```python
from build123d import *

# Parameters (mm, degrees)
SKETCH1_R           = 5
BOSS_EXTRUDE1_DEPTH = 32
SKETCH1_4_R         = 7.5
SKETCH1_4_R_2       = 5
BOSS_EXTRUDE2_DEPTH = 5
BOSS_EXTRUDE3_START = 27
SKETCH1_5_R         = 7.5
SKETCH1_5_R_2       = 5
BOSS_EXTRUDE3_DEPTH = 5


with BuildPart() as part:
    # Sketch1 → Boss-Extrude1 (new body)
    with BuildSketch(Plane.XY):
        Circle(SKETCH1_R)
    extrude(amount=BOSS_EXTRUDE1_DEPTH)

    # Sketch1<4> → Boss-Extrude2 (add)
    with BuildSketch(Plane.XY):
        Circle(SKETCH1_4_R)
        Circle(SKETCH1_4_R_2, mode=Mode.SUBTRACT)
    extrude(amount=BOSS_EXTRUDE2_DEPTH)

    # Sketch1<5> → Boss-Extrude3 (add)
    with BuildSketch(Plane.XY.offset(BOSS_EXTRUDE3_START)):
        Circle(SKETCH1_5_R)
        Circle(SKETCH1_5_R_2, mode=Mode.SUBTRACT)
    extrude(amount=BOSS_EXTRUDE3_DEPTH)


solid = part.part
```
For this review, take the finished solid that the model builds, in its own axes (mm). A direction names the side the tool comes from. Round coordinates to 2 decimals unless told otherwise and drop trailing zeros. Write each loop counter-clockwise with the first axis right and the second up, starting at its lowest first coordinate (ties: lowest second). Pieces come first, ordered by that corner, then holes. Notation, with made-up numbers: (-25.5, -5) -> (12.5, -5) arc R18 cw to (12.5, 26) -> close; hole circle Ø7 at (88.25, 22.5). An arc over 180 degrees is marked (long way). One line per question, with ' | ' between items. Start each with the question number.
(1) Add section D-D, the plane z = 24.5. Write out the cut boundary in (x, y), plus the area to 3 significant figures.
(2) Add section B-B, the plane x = 0. Write out the cut boundary in (y, z).
(3) Add section A-A, the plane y = 6. Write out the cut boundary in (x, z).
(4) Tool access review of faces 1 (the face through (2, -5, 27)), 2 (the face through (0, 0, 32)): name each direction out of +Z, -Z, +X, -X, +Y, -Y from which nothing blocks a thin tool from reaching the whole face with its end or side.
(5) For line 1 along Z through (x, y) = (5.5, 0.5); line 2 along Y through (x, z) = (-0.25, 21.5); line 3 along X through (y, z) = (1.75, 29), list the stretches that pass through material, from the lowest coordinate up. Write a range as from..to.
(6) Mouldability with a two-part tool opening along Z and no side actions: class faces 3 (the face through (0, 0, 0)), 4 (the face through (2, -5, 5)), 5 (the face through (-7.493, 0.33, 2.465)) as released by +Z, released by -Z, zero draft, split by the parting line, or undercut.
(7) Insertion check: P1, Ø4, axis at y = -2, z = 21, coming from the -X side; P2, Ø8, axis at x = -1, z = 19, coming from the +Y side; P3, Ø3, axis at x = -1.5, z = 13.5, coming from the -Y side. Each pin has a flat end and moves straight along its axis. Give the tip position at first contact, or say it passes through.
Answer list:
1) outline: circle Ø10 at (0, 0) | area: 78.5 mm²
2) outline: (-7.5, 0) -> (7.5, 0) -> (7.5, 5) -> (5, 5) -> (5, 27) -> (7.5, 27) -> (7.5, 32) -> (-7.5, 32) -> (-7.5, 27) -> (-5, 27) -> (-5, 5) -> (-7.5, 5) -> close
3) outline: (-4.5, 0) -> (4.5, 0) -> (4.5, 5) -> (-4.5, 5) -> close; (-4.5, 27) -> (4.5, 27) -> (4.5, 32) -> (-4.5, 32) -> close
4) face 1: none | face 2: +Z, +X, -X, +Y, -Y
5) line 1: 0..5, 27..32 | line 2: -4.99..4.99 | line 3: -7.29..7.29
6) face 3: released by -Z | face 4: undercut | face 5: zero draft
7) P1: x = -5 | P2: y = 5 | P3: y = -5
